```python
from build123d import *


with BuildPart() as part:
    # Эскиз1 → Повернуть1 (revolve)
    with BuildSketch(Plane(origin=(0, 0, 0), x_dir=(-1, 0, 0), z_dir=(0, 0, -1)), mode=Mode.PRIVATE) as revolve_1_sk:
        Polygon((-22, 0), (0, 0), (0, 20.07179677), (-12, 27), (-12, 59), (-10, 59), (-10, 123), (-12, 125), (-19, 125), (-19, 113), (-22, 110), (-22, 27), (-32.5, 27), (-32.5, 32), (-45, 32), (-45, 23), (-38, 23), (-38, 15), (-45, 15), (-45, 8), (-22, 8), align=None)
    revolve(revolve_1_sk.sketch.rotate(Axis((0, 0, 0), (0, 1, 0)), 180), axis=Axis((0, 0, 0), (0, 1, 0)))


solid = part.part
```
Verification items for the finished model (mm, model axes). A direction names the side the tool comes from. Coordinates: 2 decimals unless noted, no trailing zeros. Order: outer loops, then holes, each group sorted by start corner. A loop starts at its lowest first (then second) coordinate and runs counter-clockwise, first axis right, second up. Notation, with made-up numbers: (75.25, 19.25) - (100.25, 19.25) arc R8 ccw to (100.25, 29.25) - close; hole circle Ø4 at (-3, -33). An arc over 180 degrees is marked (long way). Return JSON: item names as keys, results as strings.
(1) Thickness scan on line 1 along Z through (x, y) = (0, 30); line 2 along Y through (x, z) = (-36.5, 20); line 3 along Z through (x, y) = (0, 38). Record the ranges inside material, lowest first.
Filled sheet:
{"line 1": "z = -45 to -32.5, -22 to -12, 12 to 22, 32.5 to 45", "line 2": "y = 8 to 15, 23 to 32", "line 3": "z = -22 to -12, 12 to 22"}
(2) Go/stop test with flat-tipped pins: pin 1 (4 mm diameter, centred on x = -1, y = 97, fed in from -Z); pin 2 (2 mm diameter, centred on y = 54.5, z = -8.5, fed in from -X); pin 3 (8 mm diameter, centred on x = 10, y = 42.5, fed in from +Z). Record where each tip stops, or that it passes through.
Filled sheet:
{"pin 1": "stops at z = -22", "pin 2": "stops at x = -20.68", "pin 3": "stops at z = 21.17"}
(3) Section check B-B, the plane y = 94. Record the cut outline in (x, z), and give its area (3 significant figures).
Filled sheet:
{"outline": "circle Ø44 at (0, 0); hole circle Ø20 at (0, 0)", "area": "1,210 mm^2"}
(4) Section check C-C, the plane y = 12. Record the cut outline in (x, z), and give its area (3 significant figures).
Filled sheet:
{"outline": "circle Ø90 at (0, 0)", "area": "6,360 mm^2"}
(5) Section check A-A, the plane x = 28. Record the cut outline in (y, z).
Filled sheet:
{"outline": "(8, -35.23) - (15, -35.23) - (15, -25.69) - (23, -25.69) - (23, -35.23) - (32, -35.23) - (32, -16.5) - (27, -16.5) - (27, 16.5) - (32, 16.5) - (32, 35.23) - (23, 35.23) - (23, 25.69) - (15, 25.69) - (15, 35.23) - (8, 35.23) - close"}
(6) Mould release check, pull along Z, two halves, no side actions. Record for faces 1 (the cylindrical face through (-11.446, 43.224, 3.604)), 2 (the conical face through (0.45, 21.27, -2.03)), 3 (the flat face through (0, 0, 0)), 4 (the cylindrical face through (4.119, 118.916, -18.548)): pulls with the +Z half, pulls with the -Z half, needs draft (parallel to the pull), parting line crosses it, or undercut.
Filled sheet:
{"face 1": "undercut", "face 2": "undercut", "face 3": "needs draft", "face 4": "parting line crosses it"}
(7) Section check D-D, the plane x = -27.5. Record the cut outline in (y, z).
Filled sheet:
{"outline": "(8, -35.62) - (15, -35.62) - (15, -26.22) - (23, -26.22) - (23, -35.62) - (32, -35.62) - (32, -17.32) - (27, -17.32) - (27, 17.32) - (32, 17.32) - (32, 35.62) - (23, 35.62) - (23, 26.22) - (15, 26.22) - (15, 35.62) - (8, 35.62) - close"}
(8) Access from +Z, -Z, +X, -X, +Y, -Y to the whole of each face (thin tool, end or side, straight path). Record for faces 5 (the flat face through (-9, 8, 21)), 6 (the flat face through (-37, 15, -10)), 7 (the cylindrical face through (4.769, 67.919, -21.477)), 8 (the flat face through (-0.3, 125, -12.4)).
Filled sheet:
{"face 5": "-Y", "face 6": "none", "face 7": "+Y", "face 8": "+Z, -Z, +X, -X, +Y"}
